```python
from build123d import *

# Parameters (mm, degrees)
PAD_DEPTH              = 120
SKETCH001_W            = 2.8
SKETCH001_H            = 12.5
SKETCH001_W_2          = 2.75
POCKET_DEPTH           = 1.3
POCKET001_DEPTH        = 11.75
POCKET004_DEPTH        = 14
LINEARPATTERN001_COUNT = 4
LINEARPATTERN001_PITCH = 5
LINEARPATTERN_COUNT    = 4
LINEARPATTERN_PITCH    = 5
SKETCH011_W            = 10
SKETCH011_H            = 10
POCKET005_DEPTH        = 1.5
LINEARPATTERN002_COUNT = 9
LINEARPATTERN002_PITCH = 12


with BuildPart() as part:
    # Sketch → Pad (new body)
    with BuildSketch(Plane.YZ):
        Polygon((0, 0), (0, 2), (1.990567, 3.5), (1.990567, 4.8), (2.490567, 5.3), (1.990567, 5.8), (1.990567, 8.8), (9.9, 8.8), (9.9, 0), align=None)
    extrude(amount=PAD_DEPTH)

    # Mirrored: part across face of Pad


with BuildPart() as part_1:
    add(part.part)
    add(part.part.mirror(Plane(origin=(60, 9.9, 4.4), x_dir=(-1, 0, 0), z_dir=(0, 1, 0))))

    # Sketch001 (on Face7 of Mirrored) → Pocket (cut)
    with BuildSketch(Plane.YX):
        with Locations((2.4, 18)):
            Rectangle(SKETCH001_W, SKETCH001_H)
        with Locations((7.4, 18)):
            Rectangle(SKETCH001_W, SKETCH001_H)
        with Locations((12.4, 18)):
            Rectangle(SKETCH001_W, SKETCH001_H)
        with Locations((2.375, 100)):
            Rectangle(SKETCH001_W_2, SKETCH001_H)
        with Locations((7.4, 100)):
            Rectangle(SKETCH001_W, SKETCH001_H)
        with Locations((12.4, 100)):
            Rectangle(SKETCH001_W, SKETCH001_H)
        with Locations((17.4, 18)):
            Rectangle(SKETCH001_W, SKETCH001_H)
        with Locations((17.4, 100)):
            Rectangle(SKETCH001_W, SKETCH001_H)
    extrude(amount=-POCKET_DEPTH, mode=Mode.SUBTRACT)

    # Sketch002 (on Face4 of Pocket) → Pocket001 (cut)
    with BuildSketch(Plane(origin=(0, 0, 0), x_dir=(0, 1, 0), z_dir=(-1, 0, 0))):
        Polygon((18.2, 0), (18.9, -1), (18.6, -1.3), (16.2, -1.3), (15.9, -1), (16.6, 0), align=None)
    pocket001 = extrude(amount=-POCKET001_DEPTH, mode=Mode.SUBTRACT)

    # Sketch010 (on Face14 of Pocket001) → Pocket004 (cut)
    with BuildSketch(Plane.YZ.offset(93.75)):
        Polygon((15.9, 1), (16.6, 0), (18.2, 0), (18.9, 1), (18.6, 1.3), (16.2, 1.3), align=None)
    pocket004 = extrude(amount=-POCKET004_DEPTH, mode=Mode.SUBTRACT)

    # LinearPattern001: Pocket004 ×4
    with Locations(*[(0, -i * LINEARPATTERN001_PITCH, 0) for i in range(1, LINEARPATTERN001_COUNT)]):
        add(pocket004, mode=Mode.SUBTRACT)

    # LinearPattern: Pocket001 ×4
    with Locations(*[(0, -i * LINEARPATTERN_PITCH, 0) for i in range(1, LINEARPATTERN_COUNT)]):
        add(pocket001, mode=Mode.SUBTRACT)

    # Sketch011 (on Face82 of LinearPattern) → Pocket005 (cut)
    with BuildSketch(Plane(origin=(0, 0, 8.8), x_dir=(0, -1, 0), z_dir=(0, 0, 1))):
        with Locations((-9.9, 113)):
            Rectangle(SKETCH011_W, SKETCH011_H)
    pocket005 = extrude(amount=-POCKET005_DEPTH, mode=Mode.SUBTRACT)

    # LinearPattern002: Pocket005 ×9
    with Locations(*[(-i * LINEARPATTERN002_PITCH, 0, 0) for i in range(1, LINEARPATTERN002_COUNT)]):
        add(pocket005, mode=Mode.SUBTRACT)


solid = part_1.part
```
Geometry: final body of the model. Coordinates: model frame, mm. A direction names the side the tool comes from. Round coordinates to 2 decimals unless told otherwise and drop trailing zeros. Loops run counter-clockwise (first coordinate to the right, second up) from the corner with the lowest first, then second, coordinate; pieces in that order, holes last. Notation, with made-up numbers: (-40, 73) -> (10, 73) arc R14 cw to (10, 100) -> close; hole circle Ø11 at (-20, 88.25). An arc over 180 degrees is marked (long way). Use one line per item in the form item = value. Start each with the question number.
1) Section B-B on x = 55. Output: boundary loops of the cut face in (y, z), then the cut area to 3 significant figures.
2) Draft query along Y for faces 1 (the flat face through (65, 10, 7.3)), 2 (the flat face through (120, 10, 4)), 3 (the flat face through (59.16, 0.98, 2.74)). Return one class per face: released by +Y, released by -Y, zero draft, split by the parting line, or undercut.
3) First-contact query: P1, Ø1.2, axis at x = 39, z = 7.5, coming from the +Y side; P2, Ø0.6, axis at y = 18, z = 0.5, coming from the -X side; P3, Ø1.5, axis at x = 94, z = 3.5, coming from the +Y side. Flat tips, straight axial feed; report the tip coordinate or a pass-through.
4) Line query: L1, parallel to Y at x = 82, z = 1.25; L2, parallel to Y at x = 60.5, z = 7.5; L3, parallel to Z at x = 49, y = 7.25. Output: solid intervals per line, ascending.
5) Access query for faces 4 (the flat face through (93, 17, 1.3)), 5 (the flat face through (59, 17.809, 7)), 6 (the flat face through (41, 10, 7.3)), 7 (the flat face through (59, 10, 8.8)), 8 (the flat face through (59, 1.991, 7)). Directions: +Z, -Z, +X, -X, +Y, -Y. A direction counts if a zero-diameter tool reaches every point of the face in a straight line with its end or side. Return the directions, or none.
Response:
q1.outline = (0, 0) -> (19.8, 0) -> (19.8, 2) -> (17.81, 3.5) -> (17.81, 4.8) -> (17.31, 5.3) -> (17.81, 5.8) -> (17.81, 8.8) -> (14.9, 8.8) -> (14.9, 7.3) -> (4.9, 7.3) -> (4.9, 8.8) -> (1.99, 8.8) -> (1.99, 5.8) -> (2.49, 5.3) -> (1.99, 4.8) -> (1.99, 3.5) -> (0, 2) -> close
q1.area = 135 mm^2
q2.face_1 = undercut
q2.face_2 = zero draft
q2.face_3 = released by -Y
q3.P1 = 17.81
q3.P2 = 24.25
q3.P3 = 18.8
q4.L1 = 0 to 1.15, 3.65 to 6.15, 8.65 to 11.15, 13.65 to 16.15, 18.65 to 19.8
q4.L2 = 1.99 to 4.9, 14.9 to 17.81
q4.L3 = 0 to 7.3
q5.face_4 = none
q5.face_5 = +Z, +X, -X, +Y
q5.face_6 = +Z
q5.face_7 = +Z, +X, -X, +Y, -Y
q5.face_8 = +Z, +X, -X, -Y
